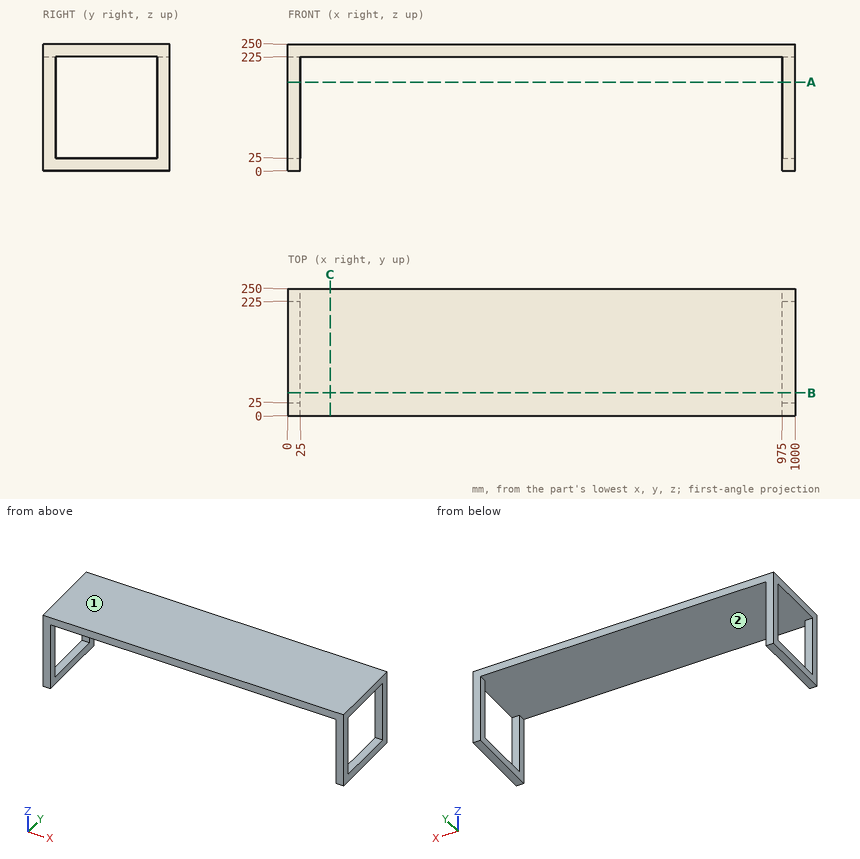
For this review, use the dimensioned drawing (mm, ordinates from the lowest corner) and the shaded views. Give positions to 0.01 mm unless a question says otherwise; leave off trailing zeros. Loops run counter-clockwise (first coordinate to the right, second up) from the corner with the lowest first, then second, coordinate; pieces in that order, holes last.
Item 1: Take a section at B-B, the plane y = 45. State the section outline as (x, z) points, and give its area (4 significant figures).
Item 2: Insertion check: pin 1 (8 mm diameter, centred on x = 486.5, y = 59, fed in from -Z); pin 2 (7.5 mm diameter, centred on x = 13.5, z = 82, fed in from -Y). Each pin has a flat end and moves straight along its axis. Give the tip position at first contact, or say it passes through.
Item 3: Take a section at C-C, the plane x = 83.5. State the section outline as (y, z) points, and give its area (3 significant figures).
Item 4: Draft analysis for pull direction X (two halves, no side actions). For the marked faces 1 and 2, state which applies: +X half, -X half, draft (parallel to the pull), parting line (faces both ways), or undercut.
Item 5: For line 1 along X through (y, z) = (202, 19); line 2 along Z through (x, y) = (819.5, 35), list the stretches that pass through material, from the lowest coordinate up.
Item 6: Take a section at A-A, the plane z = 175. State the section outline as (x, y) points, and give its area (3 significant figures).
Calculated:
1. outline: (0, 0) - (25, 0) - (25, 25) - (0, 25) - close; (0, 225) - (1000, 225) - (1000, 250) - (0, 250) - close; (975, 0) - (1000, 0) - (1000, 25) - (975, 25) - close
1. area: 26,250 mm2
2. pin 1: stops at z = 225
2. pin 2: stops at y = 0
3. outline: (0, 225) - (250, 225) - (250, 250) - (0, 250) - close
3. area: 6,250 mm2
4. face 1: draft
4. face 2: undercut
5. line 1: x = 0 to 25, 975 to 1000
5. line 2: z = 225 to 250
6. outline: (0, 0) - (25, 0) - (25, 25) - (0, 25) - close; (0, 225) - (25, 225) - (25, 250) - (0, 250) - close; (975, 0) - (1000, 0) - (1000, 25) - (975, 25) - close; (975, 225) - (1000, 225) - (1000, 250) - (975, 250) - close
6. area: 2,500 mm2
